Can you work these out from the model? Positions are in its coordinate system, mm. A direction names the side the tool comes from. Give positions to 0.01 mm unless a question says otherwise; leave off trailing zeros. Write each loop counter-clockwise with the first axis right and the second up, starting at its lowest first coordinate (ties: lowest second). Pieces come first, ordered by that corner, then holes. Notation, with made-up numbers: (21.25, 6.25) - (77.25, 6.25) arc R21 ccw to (77.25, 23.25) - close; hole circle Ø11 at (-37.75, 49). An arc over 180 degrees is marked (long way). Return JSON: item names as keys, results as strings. Group by question number.
from build123d import *

# Parameters (mm, degrees)
SKETCH1_R             = 7.47268
BOSS_EXTRUDE1_DEPTH   = 50.8
SKETCH2_W             = 14.94536
SKETCH2_H             = 25.4
BOSS_EXTRUDE2_DEPTH   = 12.95146
SKETCH3_W             = 63.40856
SKETCH3_H             = 27.21864
BOSS_EXTRUDE3_DEPTH   = 50.8
SKETCH5_W             = 11.5824
SKETCH5_H             = 38.0746
BOSS_EXTRUDE4_DEPTH   = 50.8
BOSS_EXTRUDE4_2_DEPTH = 50.8
SKETCH7_W             = 11.5824
SKETCH7_H             = 27.21864
BOSS_EXTRUDE5_DEPTH   = 50.8
SKETCH8_W             = 25.37968
SKETCH8_H             = 29.31414
BOSS_EXTRUDE6_DEPTH   = 50.8
BOSS_EXTRUDE6_2_DEPTH = 50.8
SKETCH9_W             = 11.5824
SKETCH9_H             = 29.31414
BOSS_EXTRUDE7_DEPTH   = 50.8
BOSS_EXTRUDE8_DEPTH   = 2.54
BOSS_EXTRUDE9_DEPTH   = 2.54


with BuildPart() as part:
    # Sketch1 → Boss-Extrude1 (new body)
    with BuildSketch(Plane.XY):
        Circle(SKETCH1_R)
    extrude(amount=-BOSS_EXTRUDE1_DEPTH)

    # Sketch2 → Boss-Extrude2 (add)
    with BuildSketch(Plane(origin=(0, 0, -50.8), x_dir=(-1, 0, 0), z_dir=(0, 0, -1))):
        with Locations((0, 12.7)):
            Rectangle(SKETCH2_W, SKETCH2_H)
    extrude(amount=-BOSS_EXTRUDE2_DEPTH)

    # Sketch3 → Boss-Extrude3 (add)
    with BuildSketch(Plane(origin=(0, 0, -50.8), x_dir=(-1, 0, 0), z_dir=(0, 0, -1))):
        with Locations((0, 39.00932)):
            Rectangle(SKETCH3_W, SKETCH3_H)
    extrude(amount=-BOSS_EXTRUDE3_DEPTH)



with BuildPart() as body_2:
    # Sketch5 → Boss-Extrude4 (new body)
    with BuildSketch(Plane(origin=(0, 0, -50.8), x_dir=(-1, 0, 0), z_dir=(0, 0, -1))):
        with Locations((-37.49548, 71.65594)):
            Rectangle(SKETCH5_W, SKETCH5_H)
    extrude(amount=-BOSS_EXTRUDE4_DEPTH)


with BuildPart() as body_3:
    # Sketch5 → Boss-Extrude4 2 (new body)
    with BuildSketch(Plane(origin=(0, 0, -50.8), x_dir=(-1, 0, 0), z_dir=(0, 0, -1))):
        with Locations((37.49548, 71.65594)):
            Rectangle(SKETCH5_W, SKETCH5_H)
    extrude(amount=-BOSS_EXTRUDE4_2_DEPTH)


with BuildPart() as part_1:
    add(part.part)

    add(body_2.part)  # Boss-Extrude5 merges body 2

    add(body_3.part)  # Boss-Extrude5 merges body 3
    # Sketch7 → Boss-Extrude5 (add)
    with BuildSketch(Plane(origin=(0, 0, -50.8), x_dir=(-1, 0, 0), z_dir=(0, 0, -1))):
        with Locations((-37.49548, 39.00932)):
            Rectangle(SKETCH7_W, SKETCH7_H)
        with Locations((37.49548, 39.00932)):
            Rectangle(SKETCH7_W, SKETCH7_H)
    extrude(amount=-BOSS_EXTRUDE5_DEPTH)



with BuildPart() as body_2_2:
    # Sketch8 → Boss-Extrude6 (new body)
    with BuildSketch(Plane(origin=(0, 0, -50.8), x_dir=(-1, 0, 0), z_dir=(0, 0, -1))):
        with Locations((-19.01444, 105.35031)):
            Rectangle(SKETCH8_W, SKETCH8_H)
    extrude(amount=-BOSS_EXTRUDE6_DEPTH)


with BuildPart() as body_3_2:
    # Sketch8 → Boss-Extrude6 2 (new body)
    with BuildSketch(Plane(origin=(0, 0, -50.8), x_dir=(-1, 0, 0), z_dir=(0, 0, -1))):
        with Locations((19.01444, 105.35031)):
            Rectangle(SKETCH8_W, SKETCH8_H)
    extrude(amount=-BOSS_EXTRUDE6_2_DEPTH)


with BuildPart() as part_2:
    add(part_1.part)

    add(body_2_2.part)  # Boss-Extrude7 merges body 2 2

    add(body_3_2.part)  # Boss-Extrude7 merges body 3 2
    # Sketch9 → Boss-Extrude7 (add)
    with BuildSketch(Plane(origin=(0, 0, -50.8), x_dir=(-1, 0, 0), z_dir=(0, 0, -1))):
        with Locations((-37.49548, 105.35031)):
            Rectangle(SKETCH9_W, SKETCH9_H)
        with Locations((37.49548, 105.35031)):
            Rectangle(SKETCH9_W, SKETCH9_H)
    extrude(amount=-BOSS_EXTRUDE7_DEPTH)

    # Sketch10 → Boss-Extrude8 (add)
    with BuildSketch(Plane.ZY.offset(7.47268)):
        Polygon((-37.84854, 0), (-12.44854, 25.4), (-37.84854, 25.4), align=None)
    extrude(amount=-BOSS_EXTRUDE8_DEPTH)

    # Sketch11 → Boss-Extrude9 (add)
    with BuildSketch(Plane(origin=(7.47268, 0, 0), x_dir=(0, 0, -1), z_dir=(1, 0, 0))):
        Polygon((37.84854, 0), (12.44854, 25.4), (37.84854, 25.4), align=None)
    extrude(amount=-BOSS_EXTRUDE9_DEPTH)


solid = part_2.part
1) On a 3-axis mill with a long thin cutter (end or side, diameter ignored), from which of +Z, -Z, +X, -X, +Y, -Y can I reach the whole of each face in a straight line? I mean faces 5 (the face through (-4.933, 18, -28)), 6 (the face through (-7.473, 16, -36)), 7 (the face through (31.704, 71, -26)). Say none if no direction works.
2) We'd pull the mould along X, two halves only. Please class faces 1 (the face through (0, 16, -37.849)), 2 (the face through (7.473, 16, -36)), 3 (the face through (0, 52.619, -26)), 4 (the face through (-6.22, 15.344, -22.504)): pulls with the +X half, pulls with the -X half, needs draft (parallel to the pull), parting line crosses it, or undercut.
3) Imagine slicing it at A-A, the plane y = 55. Write out the boundary of the cut face in (x, z).
4) Will these pins go through, and if not, where does the flat tip stop? pin 1 Ø12.5 at (x, z) = (13, -16.5) entering from -Y; pin 2 Ø8 at (x, z) = (-20, -6) entering from -Y; pin 3 Ø3 at (x, y) = (0, 19) entering from +Z.
5) I need wall thicknesses on line 1 along Y through (x, z) = (-31, -31); line 2 along X through (y, z) = (77.5, -1.5); line 3 along Y through (x, z) = (33, -45.5). Which ranges of each line are inside material? Lowest first, please.
6) Imagine slicing it at D-D, the plane z = -43.5. Write out the boundary of the cut face in (x, y).
7) Imagine slicing it at B-B, the plane x = -30. Write out the boundary of the cut face in (y, z).
8) Imagine slicing it at C-C, the plane z = -21. Write out the boundary of the cut face in (x, y).
Resolved:
{
 "1": {"face 5": "+Z", "face 6": "+Z, -Z, -X, -Y", "face 7": "+Z, -Z"},
 "2": {"face 1": "undercut", "face 2": "pulls with the +X half", "face 3": "undercut", "face 4": "needs draft"},
 "3": {"outline": "(-43.29, -50.8) - (-31.7, -50.8) - (-31.7, 0) - (-43.29, 0) - close; (31.7, -50.8) - (43.29, -50.8) - (43.29, 0) - (31.7, 0) - close"},
 "4": {"pin 1": "y = -3.21", "pin 2": "y = 25.4", "pin 3": "z = -37.85"},
 "5": {"line 1": "25.4 to 52.62, 90.69 to 120.01", "line 2": "-43.29 to -31.7, 31.7 to 43.29", "line 3": "25.4 to 120.01"},
 "6": {"outline": "(-43.29, 25.4) - (-7.47, 25.4) - (-7.47, 0) arc R7.47 ccw to (7.47, 0) - (7.47, 25.4) - (43.29, 25.4) - (43.29, 120.01) - (6.32, 120.01) - (6.32, 90.69) - (31.7, 90.69) - (31.7, 52.62) - (-31.7, 52.62) - (-31.7, 90.69) - (-6.32, 90.69) - (-6.32, 120.01) - (-43.29, 120.01) - close"},
 "7": {"outline": "(25.4, -50.8) - (52.62, -50.8) - (52.62, 0) - (25.4, 0) - close; (90.69, -50.8) - (120.01, -50.8) - (120.01, 0) - (90.69, 0) - close"},
 "8": {"outline": "(-43.29, 25.4) - (-7.47, 25.4) - (-7.47, 16.85) - (-4.93, 16.85) - (-4.93, 25.4) - (4.93, 25.4) - (4.93, 16.85) - (7.47, 16.85) - (7.47, 25.4) - (43.29, 25.4) - (43.29, 120.01) - (6.32, 120.01) - (6.32, 90.69) - (31.7, 90.69) - (31.7, 52.62) - (-31.7, 52.62) - (-31.7, 90.69) - (-6.32, 90.69) - (-6.32, 120.01) - (-43.29, 120.01) - close; circle Ø14.95 at (0, 0)"}
}
